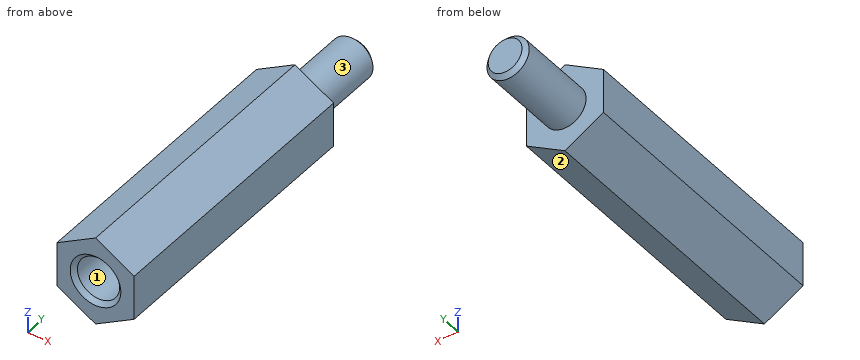
Autodesk Inventor part; units mm, degrees
ref_plane "YZ Plane" through (0, 0, 0) normal (1, 0, 0) x (0, 1, 0)
ref_plane "XZ Plane" through (0, 0, 0) normal (0, 1, 0) x (-1, 0, 0)
ref_plane "XY Plane" through (0, 0, 0) normal (0, 0, 1) x (1, 0, 0)
sketch "Sketch1" plane through (0, 0, 0) normal (0, 1, 0) x (-1, 0, 0)
  line L0 (0, 3.1639) -> (2.74, 1.5819)
  line L1 (2.74, 1.5819) -> (2.74, -1.5819)
  line L2 (2.74, -1.5819) -> (0, -3.1639)
  line L3 (0, -3.1639) -> (-2.74, -1.5819)
  line L4 (-2.74, -1.5819) -> (-2.74, 1.5819)
  line L5 (-2.74, 1.5819) -> (0, 3.1639)
  point P0 (0, 0)
  point P1 (0, 0)
  dimension "d0" = 5.48
extrude "Extrusion1" add sketch "Sketch1" along normal blind 20
sketch "Sketch2" plane through (0, 20, 0) normal (0, 1, 0) x (1, 0, 0)
  circle A0 centre (0, 0) radius 1.5
  dimension "d3" = 3
extrude "Extrusion2" add sketch "Sketch2" along normal blind 6
thread "Thread1"
chamfer "Chamfer1" distance 0.3 angle 45 1 edges at (-1.5, 26, 0)
sketch "Sketch3" plane through (0, 0, 0) normal (0, -1, 0) x (1, 0, 0)
  circle A0 centre (0, 0) radius 1.5
  dimension "d11" = 3
extrude "Extrusion3" cut sketch "Sketch3" against normal blind 7
thread "Thread2"
chamfer "Chamfer2" distance 0.3 angle 45 1 edges at (-1.5, 0, 0)
properties part number "20mm_support"
Design review of the part built by this model. Coordinates are the model's own, in mm. Face numbers are marked on the shaded views. A direction names the side the tool comes from. Give positions to 0.01 mm unless a question says otherwise; leave off trailing zeros. Loops run counter-clockwise (first coordinate to the right, second up) from the corner with the lowest first, then second, coordinate; pieces in that order, holes last. Notation, with made-up numbers: M 85.5,4 L 114.5,4 A18 ccw 114.5,39 Z; hole C -26.75,-38 d3. An arc over 180 degrees is marked long. Return JSON: item names as keys, results as strings. Group by question number.
Item 1: We need section C-C (y = 21). Give the boundary of the cut face in (x, z).
Item 2: We need section A-A (z = 0). Give the boundary of the cut face in (x, y).
Item 3: We need section B-B (y = 15.5). Give the boundary of the cut face in (x, z).
Item 4: For probe 1 along Y at (x, z) = (-0.1, 0.5); probe 2 along Y at (x, z) = (0, -2); probe 3 along Z at (x, y) = (1.3, 21.5), list the stretches that pass through material, from the lowest coordinate up.
Item 5: Insertion check: pin 1 Ø1.5 at (x, z) = (0.5, 0) entering from -Y; pin 2 Ø2.5 at (x, z) = (0.5, 0) entering from -Y; pin 3 Ø1.5 at (x, y) = (2, 19.5) entering from +Z. Each pin has a flat end and moves straight along its axis. Give the tip position at first contact, or say it passes through.
Item 6: Tool access review of the marked faces 1, 2 and 3: name each direction out of +Z, -Z, +X, -X, +Y, -Y from which nothing blocks a thin tool from reaching the whole face with its end or side.
Item 7: We need section D-D (z = -2.5). Give the boundary of the cut face in (x, y), and give its area (3 significant figures).
Output:
{
 "1": {"outline": "C 0,0 d3"},
 "2": {"outline": "M -2.74,0 L -1.8,0 L -1.5,0.3 L -1.5,7 L 1.5,7 L 1.5,0.3 L 1.8,0 L 2.74,0 L 2.74,20 L 1.5,20 L 1.5,25.7 L 1.2,26 L -1.2,26 L -1.5,25.7 L -1.5,20 L -2.74,20 Z"},
 "3": {"outline": "M -2.74,-1.58 L 0,-3.16 L 2.74,-1.58 L 2.74,1.58 L 0,3.16 L -2.74,1.58 Z"},
 "4": {"probe 1": "y = 7 to 26", "probe 2": "y = 0 to 20", "probe 3": "z = -0.75 to 0.75"},
 "5": {"pin 1": "stops at y = 7", "pin 2": "stops at y = 0.05", "pin 3": "stops at z = 2.44"},
 "6": {"face 1": "-Y", "face 2": "-Z, +X, +Y, -Y", "face 3": "+Y"},
 "7": {"outline": "M -1.15,0 L 1.15,0 L 1.15,20 L -1.15,20 Z", "area": "46.0 mm^2"}
}
